```python
from build123d import *

# Parameters (mm, degrees)
CROQUIS1_W              = 735
CROQUIS1_H              = 95
SALIENTE_EXTRUIR1_DEPTH = 1
SALIENTE_EXTRUIR2_DEPTH = 15
CROQUIS3_R              = 22.5
CORTAR_EXTRUIR1_DEPTH   = 1
CROQUIS4_R              = 22.5
CORTAR_EXTRUIR2_DEPTH   = 1
CROQUIS5_W              = 1
CROQUIS5_H              = 15
SALIENTE_EXTRUIR3_DEPTH = 15
SALIENTE_EXTRUIR4_REACH = 394.5
CROQUIS6_W              = 15
CROQUIS6_H              = 1
CORTAR_EXTRUIR3_REACH   = 18
CROQUIS8_W              = 1
CROQUIS8_H              = 95
SALIENTE_EXTRUIR5_DEPTH = 733
SALIENTE_EXTRUIR6_DEPTH = 15
CROQUIS10_R             = 1.5
SALIENTE_EXTRUIR7_DEPTH = 3.5


with BuildPart() as part:
    # Croquis1 → Saliente-Extruir1 (new body)
    with BuildSketch(Plane(origin=(0, 0, 0), x_dir=(1, 0, 0), z_dir=(0, 1, 0))):
        Rectangle(CROQUIS1_W, CROQUIS1_H)
    extrude(amount=SALIENTE_EXTRUIR1_DEPTH)

    # Croquis2 → Saliente-Extruir2 (add)
    with BuildSketch(Plane.XZ):
        Polygon((366.5, 47.5), (366.5, -46.5), (-366.5, -46.5), (-366.5, 47.5), (-367.5, 47.5), (-367.5, -47.5), (367.5, -47.5), (367.5, 47.5), align=None)
    extrude(amount=SALIENTE_EXTRUIR2_DEPTH)

    # Croquis3 → Cortar-Extruir1 (cut)
    with BuildSketch(Plane(origin=(0, 0, -47.5), x_dir=(-1, 0, 0), z_dir=(0, 0, -1))):
        with Locations((0, 10)):
            Circle(CROQUIS3_R)
    extrude(amount=-CORTAR_EXTRUIR1_DEPTH, mode=Mode.SUBTRACT)

    # Croquis4 → Cortar-Extruir2 (cut)
    with BuildSketch(Plane(origin=(0, 1, 0), x_dir=(1, 0, 0), z_dir=(0, 1, 0))):
        with Locations((0, 56.5)):
            Circle(CROQUIS4_R)
    extrude(amount=-CORTAR_EXTRUIR2_DEPTH, mode=Mode.SUBTRACT)

    # Croquis5 → Saliente-Extruir3 (add)
    with BuildSketch(Plane.XZ):
        with Locations((-25.5, -39)):
            Rectangle(CROQUIS5_W, CROQUIS5_H)
        with Locations((25.5, -39)):
            Rectangle(CROQUIS5_W, CROQUIS5_H)
    extrude(amount=SALIENTE_EXTRUIR3_DEPTH)

    # Croquis6 → Saliente-Extruir4 (add, up to next)
    with BuildSketch(Plane(origin=(-25, 0, 0), x_dir=(0, 0, -1), z_dir=(1, 0, 0)), mode=Mode.PRIVATE) as saliente_extruir4_sk1:
        with Locations((39, -14.5)):
            Rectangle(CROQUIS6_W, CROQUIS6_H)
    saliente_extruir4_tool1 = extrude(saliente_extruir4_sk1.sketch, amount=SALIENTE_EXTRUIR4_REACH, mode=Mode.PRIVATE) - part.part
    add(saliente_extruir4_tool1.solids().sort_by_distance((-25, -14.5, -39))[0])

    # Croquis7 → Cortar-Extruir3 (cut, up to next)
    with BuildSketch(Plane.XZ.offset(15), mode=Mode.PRIVATE) as cortar_extruir3_sk1:
        with BuildLine():
            Line((-6.54864521, -34.909050446), (6.54864521, -34.909050446))
            ThreePointArc((6.54864521, -34.909050446), (8.601520455, -36.961925691), (6.54864521, -39.014800936))
            Line((6.54864521, -39.014800936), (-6.54864521, -39.014800936))
            ThreePointArc((-6.54864521, -39.014800936), (-8.601520455, -36.961925691), (-6.54864521, -34.909050446))
        make_face()
    cortar_extruir3_tool1 = extrude(cortar_extruir3_sk1.sketch, amount=-CORTAR_EXTRUIR3_REACH, mode=Mode.PRIVATE) & part.part
    add(cortar_extruir3_tool1.solids().sort_by_distance((0, -15, -36.961926))[0], mode=Mode.SUBTRACT)

    # Croquis8 → Saliente-Extruir5 (add)
    with BuildSketch(Plane.ZY.offset(-366.5)):
        with Locations((47, -47.5)):
            Rectangle(CROQUIS8_W, CROQUIS8_H)
    extrude(amount=SALIENTE_EXTRUIR5_DEPTH)

    # Croquis9 → Saliente-Extruir6 (add)
    with BuildSketch(Plane(origin=(0, 0, 46.5), x_dir=(-1, 0, 0), z_dir=(0, 0, -1))):
        Polygon((-366.5, -15.890406143), (-365.5, -15.890406143), (-365.5, -94), (365.5, -94), (365.5, -15.890406143), (366.5, -15.890406143), (366.5, -95), (-366.5, -95), align=None)
    extrude(amount=SALIENTE_EXTRUIR6_DEPTH)

    # Croquis10 → Saliente-Extruir7 (add)
    with BuildSketch(Plane.ZY.offset(366.5)):
        with Locations((39.5, -89)):
            Circle(CROQUIS10_R)
    extrude(amount=SALIENTE_EXTRUIR7_DEPTH)


solid = part.part
```
Work out the finished part from the listing and answer in its coordinate system (mm). A direction names the side the tool comes from. Coordinates: 2 decimals unless noted, no trailing zeros. Loops run counter-clockwise (first coordinate to the right, second up) from the corner with the lowest first, then second, coordinate; pieces in that order, holes last.
1) For faces 1 (the flat face through (-365.5, -55, 39)), 2 (the flat face through (199, -7, -46.5)), 3 (the flat face through (0, -13, -46.5)), determine the directions among +Z, -Z, +X, -X, +Y, -Y from which every point of the face is accessible in a straight line to the end or side of a thin tool.
Results:
face 1: -Z
face 2: -Y
face 3: none
2) Consider probe 1 along Y at (x, z) = (290.5, 21); probe 2 along Z at (x, y) = (-248, -66.5); probe 3 along X at (y, z) = (-89, 33.5). Determine where each line is inside the solid, lowest interval first.
Results:
probe 1: y = 0 to 1
probe 2: z = 46.5 to 47.5
probe 3: x = -366.5 to -365.5, 365.5 to 366.5
3) Flat-ended cylindrical pins translate along their axes: pin 1 (3 mm diameter, centred on x = 220, z = -35, fed in from -Y); pin 2 (12 mm diameter, centred on y = -4, z = -39, fed in from -X); pin 3 (12 mm diameter, centred on x = -210, y = -57, fed in from -Z). Find the tip coordinate at first contact, or state that the pin passes through.
Results:
pin 1: stops at y = 0
pin 2: stops at x = -367.5
pin 3: stops at z = 46.5
4) For a pull along Z with two mould halves and no side action, classify faces 4 (the flat face through (0, -14, -41)), 5 (the cylindrical face through (-0.3, 0.5, -34)), 6 (the flat face through (5, -48, 47.5)) as +Z half, -Z half, draft (parallel to the pull), parting line (faces both ways), or undercut.
Results:
face 4: undercut
face 5: -Z half
face 6: +Z half
5) Section A-A (x = 143.5) is taken. Give the vertices of the cut face in (y, z), plus the area to 3 significant figures.
Results:
outline: (-95, 31.5) - (-94, 31.5) - (-94, 46.5) - (0, 46.5) - (0, -46.5) - (-15, -46.5) - (-15, -47.5) - (1, -47.5) - (1, 47.5) - (-95, 47.5) - close
area: 220 mm2
6) Section B-B (y = -72) is taken. Give the vertices of the cut face in (x, z), plus the area to 3 significant figures.
Results:
outline: (-366.5, 31.5) - (-365.5, 31.5) - (-365.5, 46.5) - (365.5, 46.5) - (365.5, 31.5) - (366.5, 31.5) - (366.5, 47.5) - (-366.5, 47.5) - close
area: 763 mm2
